Could you check a few things on this model? Use its own coordinates, in mm. Face numbers are marked on the shaded views. A direction names the side the tool comes from. Coordinates: 2 decimals unless noted, no trailing zeros. Loops run counter-clockwise (first coordinate to the right, second up) from the corner with the lowest first, then second, coordinate; pieces in that order, holes last.
1) For the marked faces 1, 2, 3, 4 and 5, which set-ups out of +Z, -Z, +X, -X, +Y, -Y let a thin tool reach every point of the face, with its end or its side?
2) Imagine slicing it at C-C on x = 3.25. Please give me the cut outline in (y, z).
3) Will these pins go through, and if not, where does the flat tip stop? P1, Ø2, axis at x = -0.5, z = 1.5, coming from the -Y side; P2, Ø1.5, axis at y = 0.5, z = 1, coming from the -X side; P3, Ø1.5, axis at x = -1, z = 2, coming from the +Y side.
4) Imagine slicing it at A-A on z = -0.75. Please give me the cut outline in (x, y) (3 decimals).
5) Imagine slicing it at B-B on y = 0.25. Please give me the cut outline in (x, z), plus the area to 4 significant figures.
6) If I drill on line 1 along Y through (x, z) = (0.75, 1.75); line 2 along Z through (x, y) = (3, 2.75), over which ranges is the centre line in solid material (lowest first)?
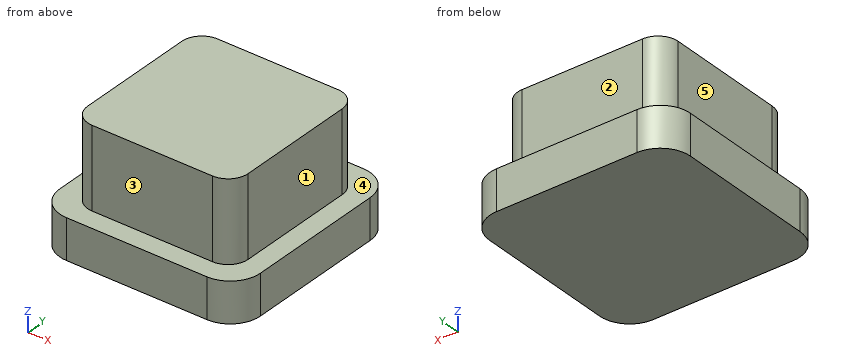
```python
from build123d import *

# Parameters (mm, degrees)
SKETCH_W     = 6
SKETCH_H     = 6
PAD_DEPTH    = 3
SKETCH001_W  = 7.5
SKETCH001_H  = 7.5
PAD001_DEPTH = 1.5
FILLET_R     = 1.125
FILLET001_R  = 0.75


with BuildPart() as part:
    # Sketch → Pad (new body)
    with BuildSketch(Plane.XY):
        Rectangle(SKETCH_W, SKETCH_H)
    extrude(amount=PAD_DEPTH)

    # Sketch001 → Pad001 (join)
    with BuildSketch(Plane.XY):
        Rectangle(SKETCH001_W, SKETCH001_H)
    extrude(amount=-PAD001_DEPTH)

    # Fillet
    fillet_edges = [part.edges().sort_by_distance(p)[0] for p in [
        (3.75, -3.75, -0.75),
        (3.75, 3.75, -0.75),
        (-3.75, 3.75, -0.75),
        (-3.75, -3.75, -0.75),
    ]]
    fillet(fillet_edges, radius=FILLET_R)

    # Fillet001
    fillet001_edges = [part.edges().sort_by_distance(p)[0] for p in [
        (3, -3, 1.5),
        (3, 3, 1.5),
        (-3, 3, 1.5),
        (-3, -3, 1.5),
    ]]
    fillet(fillet001_edges, radius=FILLET001_R)


solid = part.part
```
Filled in:
1. face 1: +Z, +X, +Y, -Y
1. face 2: +Z, +X, -X, +Y
1. face 3: +Z, +X, -X, -Y
1. face 4: +Z
1. face 5: +Z, -X, +Y, -Y
2. outline: (-3.56, -1.5) - (3.56, -1.5) - (3.56, 0) - (-3.56, 0) - close
3. P1: stops at y = -3
3. P2: stops at x = -3
3. P3: stops at y = 3
4. outline: (-3.75, -2.625) arc R1.125 ccw to (-2.625, -3.75) - (2.625, -3.75) arc R1.125 ccw to (3.75, -2.625) - (3.75, 2.625) arc R1.125 ccw to (2.625, 3.75) - (-2.625, 3.75) arc R1.125 ccw to (-3.75, 2.625) - close
5. outline: (-3.75, -1.5) - (3.75, -1.5) - (3.75, 0) - (3, 0) - (3, 3) - (-3, 3) - (-3, 0) - (-3.75, 0) - close
5. area: 29.25 mm2
6. line 1: y = -3 to 3
6. line 2: z = -1.5 to 0
